Part print with two shaded views. Sizes in mm from the minimum x, y, z corner. A direction names the side the tool comes from. Coordinates: 2 decimals unless noted, no trailing zeros. Order: outer loops, then holes, each group sorted by start corner. A loop starts at its lowest first (then second) coordinate and runs counter-clockwise, first axis right, second up. Notation, with made-up numbers: (57.5, -11) - (98.5, -11) arc R11 ccw to (98.5, 8) - close; hole circle Ø5 at (-9, 48). An arc over 180 degrees is marked (long way). Write each question's results on one line, items separated by ' | '. Start each with the question number.
Q1. Band-saw the part on A-A, the plane y = 100. Write the cut outline in (x, z).
Q2. Which spindle directions (+Z, -Z, +X, -X, +Y, -Y) get a long thin tool onto all of the face, cutting with end or side? Do the marked faces 1 and 2. Say none if no direction does.
Q3. Wall check: probe 1 along Y at (x, z) = (54, 11); probe 2 along Y at (x, z) = (32, 11) (1 decimal); probe 3 along Z at (x, y) = (5.75, 100). Give the ranges that are in metal, low to high.
Q4. Band-saw the part on C-C, the plane z = 46. Write the cut outline in (x, y), then the cut area to 3 significant figures.
Q5. Band-saw the part on B-B, the plane x = 48. Write the cut outline in (y, z), then the cut area to 3 significant figures.
Q6. Band-saw the part on D-D, the plane y = 69. Write the cut outline in (x, z), then the cut area to 3 significant figures.
Q7. Pin check, flat tips, straight feed: P1, Ø4, axis at x = 32.5, y = 72.5, coming from the +Z side; P2, Ø3, axis at y = 25.5, z = 52.5, coming from the +X side. Stop position of each tip, or through.
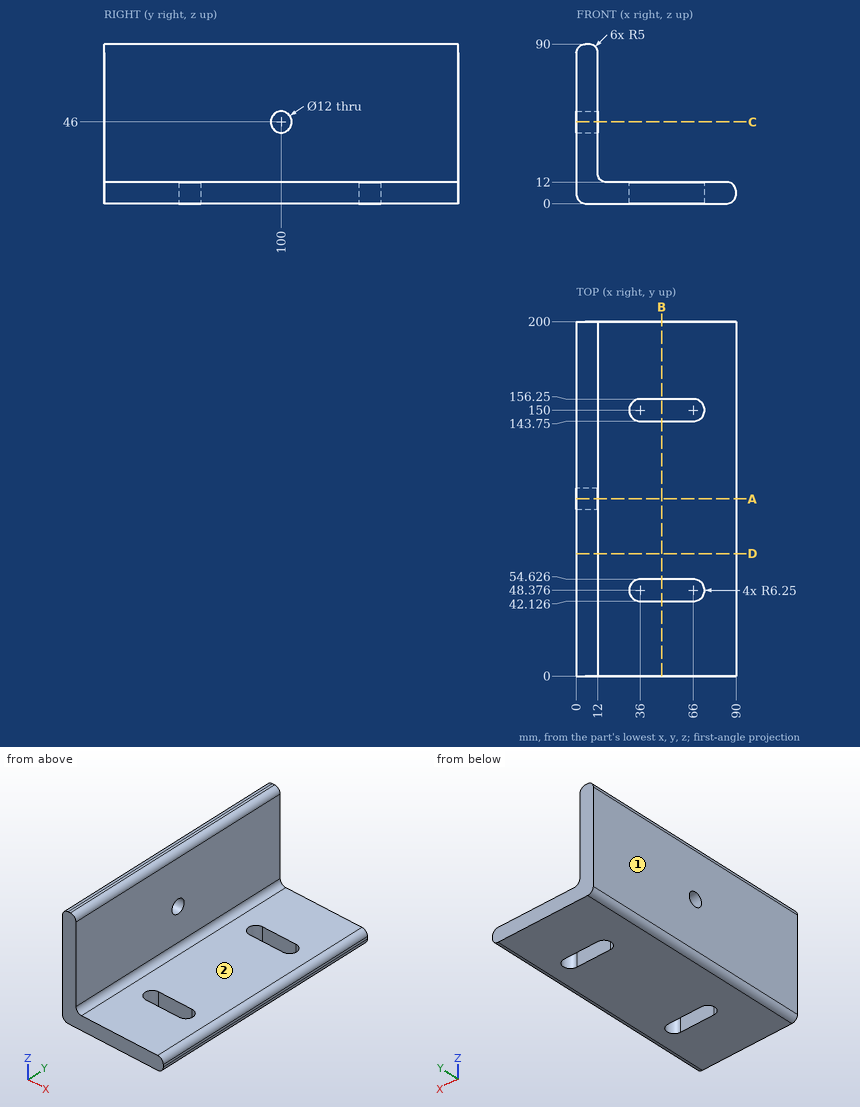
Results below:
1) outline: (0, 5) arc R5 ccw to (5, 0) - (85, 0) arc R5 ccw to (90, 5) - (90, 7) arc R5 ccw to (85, 12) - (17, 12) arc R5 cw to (12, 17) - (12, 40) - (0, 40) - close; (0, 52) - (12, 52) - (12, 85) arc R5 ccw to (7, 90) - (5, 90) arc R5 ccw to (0, 85) - close
2) face 1: +Z, -Z, -X, +Y, -Y | face 2: +Z, +X, +Y, -Y
3) probe 1: y = 0 to 42.13, 54.63 to 143.75, 156.25 to 200 | probe 2: y = 0 to 43.6, 53.2 to 145.2, 154.8 to 200 | probe 3: z = 0 to 40, 52 to 90
4) outline: (0, 0) - (12, 0) - (12, 94) - (0, 94) - close; (0, 106) - (12, 106) - (12, 200) - (0, 200) - close | area: 2,260 mm²
5) outline: (0, 0) - (42.13, 0) - (42.13, 12) - (0, 12) - close; (54.63, 0) - (143.75, 0) - (143.75, 12) - (54.63, 12) - close; (156.25, 0) - (200, 0) - (200, 12) - (156.25, 12) - close | area: 2,100 mm²
6) outline: (0, 5) arc R5 ccw to (5, 0) - (85, 0) arc R5 ccw to (90, 5) - (90, 7) arc R5 ccw to (85, 12) - (17, 12) arc R5 cw to (12, 17) - (12, 85) arc R5 ccw to (7, 90) - (5, 90) arc R5 ccw to (0, 85) - close | area: 1,990 mm²
7) P1: stops at z = 12 | P2: stops at x = 12
